For this review, take the finished solid that the model builds, in its own axes (mm). Give positions to 0.01 mm unless a question says otherwise; leave off trailing zeros. Use a Markdown table: item, result. Add a question column.
1) We need section A-A on z = -304. Give the number of separate pieces and of enclosed holes in the cut face, then the cut area to 3 significant figures.
2) Wall thickness on L1, parallel to Y at x = 11.6, z = -377; L2, parallel to X at y = 4.5, z = -236.5; L3, parallel to Y at x = 0, z = -174.5: over which ranges is each line inside the solid? List them lowest first.
3) Clearance check with flat-ended pins moving along their axes: P1, Ø1, axis at y = -14, z = -327, coming from the +X side; P2, Ø4, axis at x = 1.5, z = -206, coming from the +Y side; P3, Ø2, axis at y = -2.5, z = -204, coming from the -X side; P4, Ø6, axis at x = 3, y = 10, coming from the +Z side. State where each tip first meets the part, or that it passes through.
Autodesk Inventor part; units mm, degrees
ref_plane "C1_XY" through (0, 0, 0) normal (0, 0, 1) x (1, 0, 0)
ref_plane "C1_YZ" through (0, 0, 0) normal (1, 0, 0) x (0, 1, 0)
ref_plane "C1_ZX" through (0, 0, 0) normal (0, 1, 0) x (0, 0, 1)
sketch "Sketch_1" plane through (0, 0, 0) normal (0, 0, 1) x (1, 0, 0)
  line L0 (-15, 4) -> (-13, 4)
  line L1 (-13, 4) -> (-13, 8.25)
  line L2 (-13, 8.25) -> (-9.6642, 8.25)
  line L3 (-9.6642, 8.25) -> (-6, 4.5858)
  line L4 (-6, 4.5858) -> (-6, 0.5196)
  line L5 (-6, 0.5196) -> (-5.7, 0)
  line L6 (-5.7, 0) -> (-6, -0.5196)
  line L7 (-6, -0.5196) -> (-6, -4.5858)
  line L8 (-6, -4.5858) -> (-9.6642, -8.25)
  line L9 (-9.6642, -8.25) -> (-13, -8.25)
  line L10 (-13, -8.25) -> (-13, -4)
  line L11 (-13, -4) -> (-15, -4)
  line L12 (-15, -4) -> (-15, -13)
  arc A0 (-15, -13) -> (-13, -15) centre (-13, -13) ccw
  line L13 (-13, -15) -> (-4, -15)
  line L14 (-4, -15) -> (-4, -13)
  line L15 (-4, -13) -> (-8.25, -13)
  line L16 (-8.25, -13) -> (-8.25, -9.6642)
  line L17 (-8.25, -9.6642) -> (-4.5858, -6)
  line L18 (-4.5858, -6) -> (-0.5196, -6)
  line L19 (-0.5196, -6) -> (0, -5.7)
  line L20 (0, -5.7) -> (0.5196, -6)
  line L21 (0.5196, -6) -> (4.5858, -6)
  line L22 (4.5858, -6) -> (8.25, -9.6642)
  line L23 (8.25, -9.6642) -> (8.25, -13)
  line L24 (8.25, -13) -> (4, -13)
  line L25 (4, -13) -> (4, -15)
  line L26 (4, -15) -> (13, -15)
  arc A1 (13, -15) -> (15, -13) centre (13, -13) ccw
  line L27 (15, -13) -> (15, -4)
  line L28 (15, -4) -> (13, -4)
  line L29 (13, -4) -> (13, -8.25)
  line L30 (13, -8.25) -> (9.6642, -8.25)
  line L31 (9.6642, -8.25) -> (6, -4.5858)
  line L32 (6, -4.5858) -> (6, -0.5196)
  line L33 (6, -0.5196) -> (5.7, 0)
  line L34 (5.7, 0) -> (6, 0.5196)
  line L35 (6, 0.5196) -> (6, 4.5858)
  line L36 (6, 4.5858) -> (9.6642, 8.25)
  line L37 (9.6642, 8.25) -> (13, 8.25)
  line L38 (13, 8.25) -> (13, 4)
  line L39 (13, 4) -> (15, 4)
  line L40 (15, 4) -> (15, 13)
  arc A2 (15, 13) -> (13, 15) centre (13, 13) ccw
  line L41 (13, 15) -> (4, 15)
  line L42 (4, 15) -> (4, 13)
  line L43 (4, 13) -> (8.25, 13)
  line L44 (8.25, 13) -> (8.25, 9.6642)
  line L45 (8.25, 9.6642) -> (4.5858, 6)
  line L46 (4.5858, 6) -> (0.5196, 6)
  line L47 (0.5196, 6) -> (0, 5.7)
  line L48 (0, 5.7) -> (-0.5196, 6)
  line L49 (-0.5196, 6) -> (-4.5858, 6)
  line L50 (-4.5858, 6) -> (-8.25, 9.6642)
  line L51 (-8.25, 9.6642) -> (-8.25, 13)
  line L52 (-8.25, 13) -> (-4, 13)
  line L53 (-4, 13) -> (-4, 15)
  line L54 (-4, 15) -> (-13, 15)
  arc A3 (-13, 15) -> (-15, 13) centre (-13, 13) ccw
  line L55 (-15, 13) -> (-15, 4)
extrude "Extrusion1" add sketch "Sketch_1" against normal blind 500
sketch "Sketch2" plane through (0, 0, -500) normal (0, 0, -1) x (-1, 0, 0)
  point P0 (0, 0)
hole "Hole1" at (0, 0, -500) direction (0, 0, 1) diameter 6.8 depth 500
sketch "Sketch3" plane through (0, 0, -500) normal (0, 0, -1) x (-1, 0, 0)
  point P0 (-11.6, 11.6)
hole "Hole2" at (11.6, 11.6, -500) direction (0, 0, 1) diameter 4.2 depth 500
pattern_linear "Rectangular Pattern1" count 2 spacing 23.2 along (-1, 0, 0) count 2 spacing 23.2 along (0, -1, 0) of "Hole2"
ref_plane "C1_XY" through (0, 0, 0) normal (0, 0, 1) x (1, 0, 0)
ref_plane "C1_YZ" through (0, 0, 0) normal (1, 0, 0) x (0, 1, 0)
ref_plane "C1_ZX" through (0, 0, 0) normal (0, 1, 0) x (0, 0, 1)
ref_plane "to_frame_cap1_XY" through (0, 0, 0) normal (0, 0, 1) x (1, 0, 0)
ref_plane "to_frame_cap1_YZ" through (0, 0, 0) normal (1, 0, 0) x (0, 1, 0)
ref_plane "to_frame_cap1_ZX" through (0, 0, 0) normal (0, 1, 0) x (0, 0, 1)
ref_plane "to_frame_cap2_XY" through (0, 0, -500) normal (0, 0, -1) x (1, 0, 0)
ref_plane "to_frame_cap2_YZ" through (0, 0, -500) normal (1, 0, 0) x (0, -1, 0)
ref_plane "to_frame_cap2_ZX" through (0, 0, -500) normal (0, -1, 0) x (0, 0, -1)
properties part number "HFS6-3030-500"
Checked values:
| question | item | result |
|---|---|---|
| 1 | separate pieces | 1 |
| 1 | enclosed holes | 5 |
| 1 | area | 332 mm² |
| 2 | L1 | -15 to -13.7, -9.5 to -8.25, 8.25 to 9.5, 13.7 to 15 |
| 2 | L2 | -15 to -13, -6 to 6, 13 to 15 |
| 2 | L3 | -5.7 to -3.4, 3.4 to 5.7 |
| 3 | P1 | x = 14.94 |
| 3 | P2 | y = 6 |
| 3 | P3 | x = -6 |
| 3 | P4 | through |
